```python
from build123d import *

# Parameters (mm, degrees)
RESSALTO_EXTRUS_O1_DEPTH                            = 25
ESCAREADO_PARA_PARAFUSO_ALLEN_SEXTAVADO_D           = 13.5
ESCAREADO_PARA_PARAFUSO_ALLEN_SEXTAVADO_DEPTH       = 25
ESCAREADO_PARA_PARAFUSO_ALLEN_SEXTAVADO_CSINK_D     = 26.88
ESCAREADO_PARA_PARAFUSO_ALLEN_SEXTAVADO_CSINK_ANGLE = 90
ESCAREADO_PARA_PARAFUSO_ALLEN_SEXTAVADO_TIP         = 4.055809178
FURO_ROSCADO_DE_M121_AT_2_COUNT                     = 2
FURO_ROSCADO_DE_M121_AT_2_PITCH                     = 42
FILETE1_R                                           = 8


with BuildPart() as part:
    # Esboço1 → Ressalto-extrusão1 (new body)
    with BuildSketch(Plane.XY):
        Polygon((-25, 120), (500, 120), (525, 120), (525, 0), (500, 0), (-25, 0), (-50, 0), (-50, 120), align=None)
    extrude(amount=RESSALTO_EXTRUS_O1_DEPTH)

    # Escareado para parafuso Allen sextavado escareado de M121
    with Locations(Plane.XY.offset(25)):
        with Locations((-12.5, 102), (-12.5, 60), (-12.5, 18), (487.5, 102), (487.5, 60), (487.5, 18)):
            CounterSinkHole(ESCAREADO_PARA_PARAFUSO_ALLEN_SEXTAVADO_D / 2, ESCAREADO_PARA_PARAFUSO_ALLEN_SEXTAVADO_CSINK_D / 2, depth=ESCAREADO_PARA_PARAFUSO_ALLEN_SEXTAVADO_DEPTH, counter_sink_angle=ESCAREADO_PARA_PARAFUSO_ALLEN_SEXTAVADO_CSINK_ANGLE)
            with Locations((0, 0, -(ESCAREADO_PARA_PARAFUSO_ALLEN_SEXTAVADO_DEPTH + ESCAREADO_PARA_PARAFUSO_ALLEN_SEXTAVADO_TIP / 2))):  # 118° drill point
                Cone(0, ESCAREADO_PARA_PARAFUSO_ALLEN_SEXTAVADO_D / 2, ESCAREADO_PARA_PARAFUSO_ALLEN_SEXTAVADO_TIP, mode=Mode.SUBTRACT)

    # Esboço6 → Furo roscado de M121 (revolve, cut)
    with BuildSketch(Plane(origin=(-50, 81, 12.5), x_dir=(0, 0, 1), z_dir=(0, 1, 0))):
        Polygon((0, 0), (0, 53.064389157), (5.1, 50), (5.1, 0), align=None)
    furo_roscado_de_m121 = revolve(axis=Axis((-56.35, 81, 12.5), (1, 0, 0)), mode=Mode.SUBTRACT)

    # Furo roscado de M121 at 2: Furo roscado de M121 ×2
    with Locations(*[(0, -i * FURO_ROSCADO_DE_M121_AT_2_PITCH, 0) for i in range(1, FURO_ROSCADO_DE_M121_AT_2_COUNT)]):
        add(furo_roscado_de_m121, mode=Mode.SUBTRACT)

    # Espelhar1: Furo roscado de M121 across plane
    add(furo_roscado_de_m121.mirror(Plane.ZY.offset(-237.5)), mode=Mode.SUBTRACT)

    # Espelhar1 copy 1 sketch → Espelhar1 copy 1 (revolve, cut)
    with BuildSketch(Plane(origin=(525, 39, 12.5), x_dir=(0, 0, 1), z_dir=(0, 1, 0))):
        Polygon((0, 0), (0, -53.064389157), (5.1, -50), (5.1, 0), align=None)
    revolve(axis=Axis((531.35, 39, 12.5), (1, 0, 0)), mode=Mode.SUBTRACT)

    # Filete1
    # the kernel refuses this fillet: 8 mm, written as the material it takes off along each edge
    with BuildSketch(Plane(origin=(-50, -20, 0), x_dir=(0, 0, 1), z_dir=(0, 1, 0)), Plane(origin=(525, 140, 0), x_dir=(0, 0, 1), z_dir=(0, -1, 0))) as filete1_piece_1:
        with BuildLine():
            CenterArc((FILETE1_R, FILETE1_R), FILETE1_R, 180, 90)
            Line((0, FILETE1_R), (0, 0))
            Line((0, 0), (FILETE1_R, 0))
        make_face()
    extrude(amount=160, mode=Mode.SUBTRACT)


solid = part.part
```
Geometry check sheet. Reference: the model listing, model coordinates, mm. A direction names the side the tool comes from. Coordinates: 2 decimals unless noted, no trailing zeros. Write each loop counter-clockwise with the first axis right and the second up, starting at its lowest first coordinate (ties: lowest second). Pieces come first, ordered by that corner, then holes. Notation, with made-up numbers: M 24,3.5 L 32,3.5 A12 ccw 32,23.5 Z; hole C 88.5,-30 d6. An arc over 180 degrees is marked long. One line per item, written item: value. Start each with the question number.
(1) Sectioned sample at B-B, the plane y = 60. Enter the section's corners in (x, z), and give its area (3 significant figures).
(2) Sectioned sample at A-A, the plane x = 487.5. Enter the section's corners in (y, z), and give its area (3 significant figures).
(3) Scan lines: line 1 along Y through (x, z) = (-12.5, 5.25); line 2 along X through (y, z) = (102, 14.5); line 3 along Z through (x, y) = (-28, 81). Record each from-to range of solid material in increasing order. Write a range as [from, to].
(4) Release check for a two-part mould opening along Z. For faces 1 (the face through (481.062, 62.028, 9.027)), 2 (the face through (2.532, 39.865, 12.308)), 3 (the face through (488.42, 67.01, 18.63)) record: released by +Z, released by -Z, zero draft, split by the parting line, or undercut.
(5) Tool access check on faces 4 (the face through (-25.35, 76.7, 15.24)), 5 (the face through (481.062, 104.028, 9.027)), 6 (the face through (500.35, 76.7, 15.24)). Record the directions out of +Z, -Z, +X, -X, +Y, -Y that give a thin tool (end or side, any length) a straight path to the whole face; none if there is none.
(6) Depth check by flat-ended pin: pin 1 (12 mm diameter, centred on x = -12.5, y = 60, fed in from -Z); pin 2 (3 mm diameter, centred on x = 79.5, y = 43, fed in from -Z); pin 3 (8 mm diameter, centred on y = 81, z = 12.5, fed in from +X); pin 4 (21.5 mm diameter, centred on x = -12.5, y = 102, fed in from +Z). Enter the tip coordinate at first touch or a pass-through.
Filled sheet:
1. outline: M -50,8 A8 ccw -42,0 L -19.25,0 L -19.25,18.31 L -25.94,25 L -50,25 Z; M -5.75,0 L 480.75,0 L 480.75,18.31 L 474.06,25 L 0.94,25 L -5.75,18.31 Z; M 494.25,0 L 517,0 A8 ccw 525,8 L 525,25 L 500.94,25 L 494.25,18.31 Z
1. area: 13,600 mm²
2. outline: M 0,0 L 11.25,0 L 11.25,18.31 L 4.56,25 L 0,25 Z; M 24.75,0 L 53.25,0 L 53.25,18.31 L 46.56,25 L 31.44,25 L 24.75,18.31 Z; M 66.75,0 L 95.25,0 L 95.25,18.31 L 88.56,25 L 73.44,25 L 66.75,18.31 Z; M 108.75,0 L 120,0 L 120,25 L 115.44,25 L 108.75,18.31 Z; hole C 39,12.5 d10.2; hole C 81,12.5 d10.2
2. area: 1,690 mm²
3. line 1: [0, 11.25], [24.75, 53.25], [66.75, 95.25], [108.75, 120]
3. line 2: [-50, -19.25], [-5.75, 480.75], [494.25, 525]
3. line 3: [0, 7.4], [17.6, 25]
4. face 1: zero draft
4. face 2: undercut
4. face 3: released by +Z
5. face 4: -X
5. face 5: +Z, -Z
5. face 6: +X
6. pin 1: through
6. pin 2: z = 0
6. pin 3: x = 474.34
6. pin 4: z = 22.31
